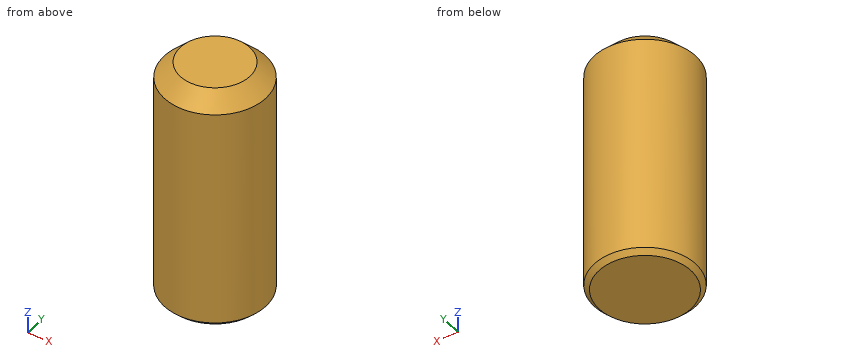
```python
from build123d import *

# Parameters (mm, degrees)
SKETCH022_R     = 3.175
PAD011_DEPTH    = 15
CHAMFER_SIZE    = 0.3
CHAMFER001_SIZE = 1


with BuildPart() as part:
    # Sketch022 → Pad011 (new body)
    with BuildSketch(Plane.XY):
        Circle(SKETCH022_R)
    extrude(amount=PAD011_DEPTH)

    # Chamfer
    chamfer_edges = [part.edges().sort_by_distance(p)[0] for p in [
        (-3.175, 0, 0),
    ]]
    chamfer(chamfer_edges, length=CHAMFER_SIZE)

    # Chamfer001
    chamfer001_edges = [part.edges().sort_by_distance(p)[0] for p in [
        (-3.175, 0, 15),
    ]]
    chamfer(chamfer001_edges, length=CHAMFER001_SIZE)


with BuildPart() as part_1:
    # Body003003 placement: moved
    add(part.part.moved(Location((0, 0, 8))))


solid = part_1.part
```
Check sheet for the modelled part. Datum: model origin and axes. Units: mm. Give positions to 0.01 mm unless a question says otherwise; leave off trailing zeros. Write each loop counter-clockwise with the first axis right and the second up, starting at its lowest first coordinate (ties: lowest second). Pieces come first, ordered by that corner, then holes.
Item 1: Scan lines: L1, parallel to Z at x = -2, y = -2; L2, parallel to Y at x = -1.25, z = 10.5; L3, parallel to Z at x = -1.5, y = -2 (3 decimals). Record each from-to range of solid material in increasing order.
Item 2: Cross-section at A-A (z = 13.5). Enter the section's corners in (x, y) (3 decimals), and give its area (3 significant figures).
Item 3: Gauge pin test, flat end, axial feed: pin 1 (2 mm diameter, centred on x = -1.5, z = 19.5, fed in from +Y). Record the tip position at first contact, or that the pin passes through.
Report:
1. L1: z = 8 to 22.35
1. L2: y = -2.92 to 2.92
1. L3: z = 8 to 22.675
2. outline: circle Ø6.35 at (0, 0)
2. area: 31.7 mm2
3. pin 1: stops at y = 3.14
